```python
from build123d import *

# Parameters (mm, degrees)
SKETCH1_R           = 3.175
BOSS_EXTRUDE1_DEPTH = 3.175
SKETCH2_R           = 3.2004
SKETCH2_R_2         = 2.4384
SKETCH2_R_3         = 3.175
CUT_EXTRUDE2_DEPTH  = 205.115710138
SKETCH3_R           = 4.73075
CUT_EXTRUDE3_DEPTH  = 1.5875


with BuildPart() as part:
    # Sketch1 → Boss-Extrude1 (new body)
    with BuildSketch(Plane(origin=(0, 0, 0), x_dir=(0, 0, -1), z_dir=(1, 0, 0))):
        with BuildLine():
            Line((12.7, 19.05), (0, 19.05))
            ThreePointArc((0, 19.05), (-19.05, 0), (0, -19.05))
            Line((0, -19.05), (12.7, -19.05))
            Line((12.7, -19.05), (12.7, -15.875))
            Line((12.7, -15.875), (25.4, -15.875))
            Line((25.4, -15.875), (25.4, -19.05))
            Line((25.4, -19.05), (38.1, -19.05))
            Line((38.1, -19.05), (38.1, -15.875))
            Line((38.1, -15.875), (50.8, -15.875))
            Line((50.8, -15.875), (50.8, -19.05))
            Line((50.8, -19.05), (63.5, -19.05))
            Line((63.5, -19.05), (63.5, -15.875))
            Line((63.5, -15.875), (76.2, -15.875))
            Line((76.2, -15.875), (76.2, -19.05))
            Line((76.2, -19.05), (88.9, -19.05))
            Line((88.9, -19.05), (88.9, -15.875))
            Line((88.9, -15.875), (101.6, -15.875))
            Line((101.6, -15.875), (101.6, -19.05))
            Line((101.6, -19.05), (114.3, -19.05))
            Line((114.3, -19.05), (114.3, -15.875))
            Line((114.3, -15.875), (127, -15.875))
            Line((127, -15.875), (127, -19.05))
            Line((127, -19.05), (139.7, -19.05))
            Line((139.7, -19.05), (139.7, -15.875))
            Line((139.7, -15.875), (152.4, -15.875))
            Line((152.4, -15.875), (152.4, -19.05))
            Line((152.4, -19.05), (165.1, -19.05))
            Line((165.1, -19.05), (165.1, -15.875))
            Line((165.1, -15.875), (177.8, -15.875))
            Line((177.8, -15.875), (177.8, -19.05))
            Line((177.8, -19.05), (190.5, -19.05))
            Line((190.5, -19.05), (190.5, -15.875))
            Line((190.5, -15.875), (203.2, -15.875))
            Line((203.2, -15.875), (203.2, 15.875))
            Line((203.2, 15.875), (190.5, 15.875))
            Line((190.5, 15.875), (190.5, 19.05))
            Line((190.5, 19.05), (177.8, 19.05))
            Line((177.8, 19.05), (177.8, 15.875))
            Line((177.8, 15.875), (165.1, 15.875))
            Line((165.1, 15.875), (165.1, 19.05))
            Line((165.1, 19.05), (152.4, 19.05))
            Line((152.4, 19.05), (152.4, 15.875))
            Line((152.4, 15.875), (139.7, 15.875))
            Line((139.7, 15.875), (139.7, 19.05))
            Line((139.7, 19.05), (127, 19.05))
            Line((127, 19.05), (127, 15.875))
            Line((127, 15.875), (114.3, 15.875))
            Line((114.3, 15.875), (114.3, 19.05))
            Line((114.3, 19.05), (101.6, 19.05))
            Line((101.6, 19.05), (101.6, 15.875))
            Line((101.6, 15.875), (88.9, 15.875))
            Line((88.9, 15.875), (88.9, 19.05))
            Line((88.9, 19.05), (76.2, 19.05))
            Line((76.2, 19.05), (76.2, 15.875))
            Line((76.2, 15.875), (63.5, 15.875))
            Line((63.5, 15.875), (63.5, 19.05))
            Line((63.5, 19.05), (50.8, 19.05))
            Line((50.8, 19.05), (50.8, 15.875))
            Line((50.8, 15.875), (38.1, 15.875))
            Line((38.1, 15.875), (38.1, 19.05))
            Line((38.1, 19.05), (25.4, 19.05))
            Line((25.4, 19.05), (25.4, 15.875))
            Line((25.4, 15.875), (12.7, 15.875))
            Line((12.7, 15.875), (12.7, 19.05))
        make_face()
        Circle(SKETCH1_R, mode=Mode.SUBTRACT)
    extrude(amount=BOSS_EXTRUDE1_DEPTH)

    # Sketch2 → Cut-Extrude2 (cut, through all)
    with BuildSketch(Plane(origin=(3.175, 0, 0), x_dir=(0, 0, -1), z_dir=(1, 0, 0))):
        with Locations((15.875, 0)):
            Circle(SKETCH2_R)
        with Locations((187.325, 0)):
            Circle(SKETCH2_R_2)
        with Locations((42.8625, -9.647e-06)):
            Circle(SKETCH2_R_3)
        with Locations((77.7875, 0)):
            Circle(SKETCH2_R_3)
    extrude(amount=-CUT_EXTRUDE2_DEPTH, mode=Mode.SUBTRACT)

    # Sketch3 → Cut-Extrude3 (cut)
    with BuildSketch(Plane(origin=(3.175, 0, 0), x_dir=(0, 0, -1), z_dir=(1, 0, 0))):
        with Locations((15.875, 0)):
            Circle(SKETCH3_R)
    extrude(amount=-CUT_EXTRUDE3_DEPTH, mode=Mode.SUBTRACT)


solid = part.part
```
Input: part model. Units: mm. Frame: model coordinates. A direction names the side the tool comes from. Coordinates: 2 decimals unless noted, no trailing zeros. Answer in a Markdown table with one row per item.
(1) Material intervals for L1, parallel to Y at x = 1.1, z = 0 (3 decimals); L2, parallel to Z at x = 2.2, y = -2; L3, parallel to Y at x = 1.45, z = -95 (3 decimals), sorted ascending. Write a range as from..to.
Model answer:
| item | result |
|---|---|
| L1 | y = -19.05..-3.175, 3.175..19.05 |
| L2 | z = -203.2..-188.72, -185.93..-80.25, -75.32..-45.33, -40.4..-20.16, -11.59..-2.47, 2.47..18.94 |
| L3 | y = -15.875..15.875 |
(2) Set-up query: faces 1 (the face through (2.39, 0.21, -11.15)), 2 (the face through (1.61, 0.95, -45.89)). Return all of +Z, -Z, +X, -X, +Y, -Y with unobstructed straight access to the full face (end or side cutting, diameter ignored); none if empty.
Model answer:
| item | result |
|---|---|
| face 1 | +X |
| face 2 | +X, -X |
(3) Mould query, pull axis Y, two halves, no side actions, for faces 3 (the face through (1.565, 0.419, 19.045)), 4 (the face through (0, 0, -91)), 5 (the face through (0.805, 0.141, -12.678)). Classes: pulls with the +Y half, pulls with the -Y half, needs draft (parallel to the pull), parting line crosses it, or undercut.
Model answer:
| item | result |
|---|---|
| face 3 | parting line crosses it |
| face 4 | needs draft |
| face 5 | undercut |
(4) Pin query (flat end, axial travel): P1, Ø1.6, axis at x = 2, y = -17, coming from the -Z side; P2, Ø1, axis at x = 1, z = -197, coming from the +Y side (3 decimals); P3, Ø1.6, axis at x = 1.5, z = -174, coming from the -Y side (3 decimals). Return the tip coordinate at first contact, or that it passes through.
Model answer:
| item | result |
|---|---|
| P1 | stops at z = -190.5 |
| P2 | stops at y = 15.875 |
| P3 | stops at y = -15.875 |
